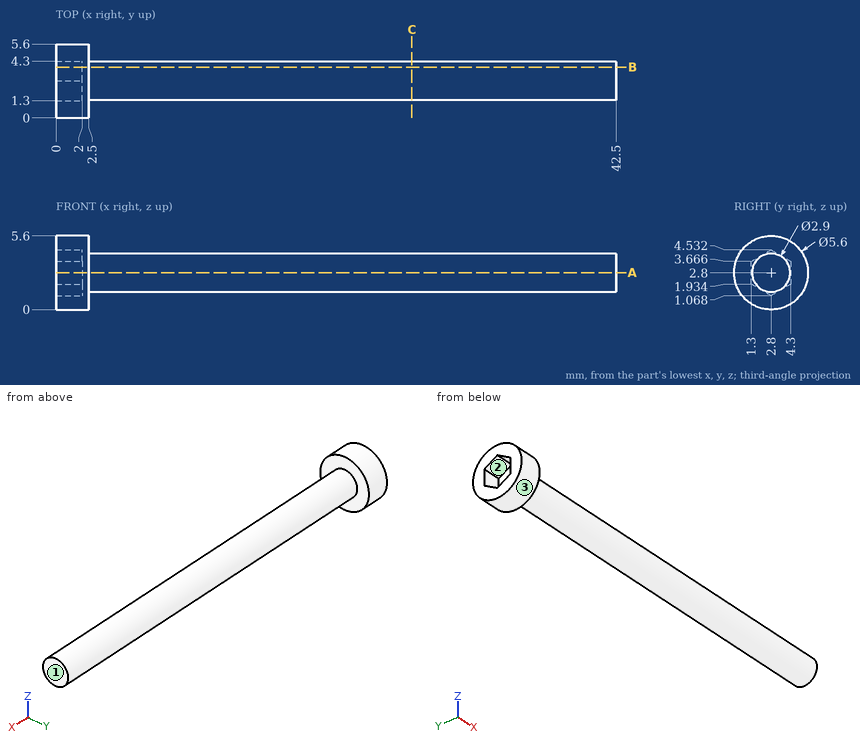
Study the drawing (mm; zero at the part's minimum x, y, z) and answer. Give positions to 0.01 mm unless a question says otherwise; leave off trailing zeros. Write each loop counter-clockwise with the first axis right and the second up, starting at its lowest first coordinate (ties: lowest second). Pieces come first, ordered by that corner, then holes. Notation, with made-up numbers: (-25, -10.5) -> (14, -10.5) arc R30 ccw to (14, 15.5) -> close; hole circle Ø8 at (-22.5, -13.75). An arc over 180 degrees is marked (long way). Answer as a JSON object with one key per item and string values. Group by question number.
1) The mould has two halves that part along Y. Classify the marked faces 1, 2 and 3: +Y half, -Y half, draft (parallel to the pull), parting line (faces both ways), or undercut.
2) Consider L1, parallel to Y at x = 12, z = 2.85; L2, parallel to X at y = 4.7, z = 1.95; L3, parallel to X at y = 3.7, z = 2.6. Determine where each line is inside the solid, lowest interval first. Write a range as from..to.
3) Find section B-B (y = 3.85). Write down the section's boundary in (x, z).
4) Find section A-A (z = 2.8). Write down the section's boundary in (x, y), and give its area (3 significant figures).
5) Find section C-C (x = 27). Write down the section's boundary in (y, z).
6) Each of these flat-tipped pins is pushed along its axis until it touches: P1, Ø1.5, axis at x = 18, y = 4.5, coming from the +Z side; P2, Ø1.5, axis at x = 25.5, z = 4, coming from the +Y side. Where does it stop, or does it pass through?
Values follow:
{
 "1": {"face 1": "draft", "face 2": "undercut", "face 3": "parting line"},
 "2": {"L1": "y = 1.35..4.25", "L2": "x = 0..2.5", "L3": "x = 2..42.5"},
 "3": {"outline": "(0, 0.2) -> (2.5, 0.2) -> (2.5, 1.8) -> (42.5, 1.8) -> (42.5, 3.8) -> (2.5, 3.8) -> (2.5, 5.4) -> (0, 5.4) -> (0, 3.93) -> (2, 3.93) -> (2, 1.67) -> (0, 1.67) -> close"},
 "4": {"outline": "(0, 0) -> (2.5, 0) -> (2.5, 1.35) -> (42.5, 1.35) -> (42.5, 4.25) -> (2.5, 4.25) -> (2.5, 5.6) -> (0, 5.6) -> (0, 4.3) -> (2, 4.3) -> (2, 1.3) -> (0, 1.3) -> close", "area": "124 mm2"},
 "5": {"outline": "circle Ø2.9 at (2.8, 2.8)"},
 "6": {"P1": "stops at z = 3.9", "P2": "stops at y = 4.18"}
}
